Design review of the part built by this model. Coordinates are the model's own, in mm. A direction names the side the tool comes from. Coordinates: 2 decimals unless noted, no trailing zeros. Write each loop counter-clockwise with the first axis right and the second up, starting at its lowest first coordinate (ties: lowest second). Pieces come first, ordered by that corner, then holes. Notation, with made-up numbers: (76.5, 47) -> (117.5, 47) arc R28 cw to (117.5, 65) -> close; hole circle Ø6 at (56, 88). An arc over 180 degrees is marked (long way). One line per question, with ' | ' between items. Start each with the question number.
Q1. Add section D-D on z = 9. State the section outline as (x, y) points.
Q2. Add section A-A on y = 0. State the section outline as (x, z) points.
Q3. Add section B-B on y = -16. State the section outline as (x, z) points.
Q4. Wall thickness on probe 1 along Y at (x, z) = (0, 4); probe 2 along Z at (x, y) = (-4, 16.5); probe 3 along X at (y, z) = (2, 2): over which ranges is each line inside the solid? List them lowest first.
Q5. For P1, Ø1.5, axis at y = 4, z = 23.5, coming from the +X side; P2, Ø6, axis at y = 1.5, z = 21, coming from the -X side; P3, Ø4, axis at x = 6, y = -1, coming from the +Z side, all flat-tipped, find the tip position at first contact; note any pin that passes through.
Q6. For faces 4 (the cylindrical face through (-0.54, -17.44, 2.54)), 5 (the cylindrical face through (-7.493, 0.33, 11.902)), list the 3-axis set-ups (+Z, -Z, +X, -X, +Y, -Y) from which the entire face can be reached by the end or side of a thin tool; tool diameter is ignored.
Q7. Add section C-C on x = -15. State the section outline as (y, z) points, and give its area (3 significant figures).
Q8. Draft analysis for pull direction X (two halves, no side actions). For faces 1 (the flat face through (3, -3, 19)), 2 (the cylindrical face through (-0.867, -3.905, 28.86)), 3 (the cylindrical face through (12.5, 0.1, 2.5)), state which applies: pulls with the +X half, pulls with the -X half, needs draft (parallel to the pull), parting line crosses it, or undercut.
from build123d import *

# Parameters (mm, degrees)
SKETCH1_R           = 20
BOSS_EXTRUDE1_DEPTH = 5
SKETCH2_R           = 7.5
BOSS_EXTRUDE2_DEPTH = 14
SKETCH3_R           = 4
BOSS_EXTRUDE3_DEPTH = 20
SKETCH4_R           = 2.5
CUT_EXTRUDE1_DEPTH  = 20


with BuildPart() as part:
    # Sketch1 → Boss-Extrude1 (new body)
    with BuildSketch(Plane.XY):
        Circle(SKETCH1_R)
    extrude(amount=BOSS_EXTRUDE1_DEPTH)

    # Sketch2 → Boss-Extrude2 (add)
    with BuildSketch(Plane.XY.offset(5)):
        Circle(SKETCH2_R)
    extrude(amount=BOSS_EXTRUDE2_DEPTH)

    # Sketch3 → Boss-Extrude3 (add)
    with BuildSketch(Plane.XY.offset(19)):
        Circle(SKETCH3_R)
    extrude(amount=BOSS_EXTRUDE3_DEPTH)

    # Sketch4 → Cut-Extrude1 (cut)
    with BuildSketch(Plane.XY.offset(5)):
        with Locations((0, 15)):
            Circle(SKETCH4_R)
        with Locations((15, 0)):
            Circle(SKETCH4_R)
        with Locations((0, -15)):
            Circle(SKETCH4_R)
        with Locations((-15, 0)):
            Circle(SKETCH4_R)
    extrude(amount=-CUT_EXTRUDE1_DEPTH, mode=Mode.SUBTRACT)


solid = part.part
Output values:
1) outline: circle Ø15 at (0, 0)
2) outline: (-20, 0) -> (-17.5, 0) -> (-17.5, 5) -> (-20, 5) -> close; (-12.5, 0) -> (12.5, 0) -> (12.5, 5) -> (7.5, 5) -> (7.5, 19) -> (4, 19) -> (4, 39) -> (-4, 39) -> (-4, 19) -> (-7.5, 19) -> (-7.5, 5) -> (-12.5, 5) -> close; (17.5, 0) -> (20, 0) -> (20, 5) -> (17.5, 5) -> close
3) outline: (-12, 0) -> (-2.29, 0) -> (-2.29, 5) -> (-12, 5) -> close; (2.29, 0) -> (12, 0) -> (12, 5) -> (2.29, 5) -> close
4) probe 1: y = -20 to -17.5, -12.5 to 12.5, 17.5 to 20 | probe 2: z = 0 to 5 | probe 3: x = -19.9 to -16.5, -13.5 to 13.5, 16.5 to 19.9
5) P1: stops at x = 2.33 | P2: stops at x = -7.5 | P3: stops at z = 19
6) face 4: +Z, -Z | face 5: +Z
7) outline: (-13.23, 0) -> (-2.5, 0) -> (-2.5, 5) -> (-13.23, 5) -> close; (2.5, 0) -> (13.23, 0) -> (13.23, 5) -> (2.5, 5) -> close | area: 107 mm2
8) face 1: needs draft | face 2: parting line crosses it | face 3: undercut
